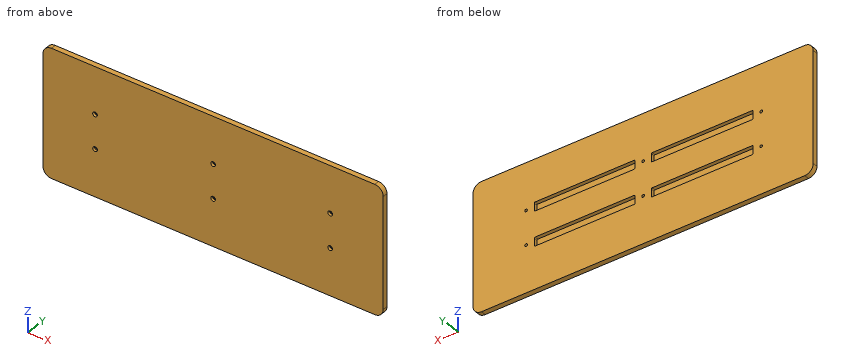
from build123d import *

# Parameters (mm, degrees)
IZIM1_W                     = 400
IZIM1_H                     = 150
Y_KSEKLIK_EKSTR_ZYON1_DEPTH = 6
IZIM2_W                     = 119.6
IZIM2_H                     = 10.4
IZIM2_W_2                   = 118.39
KES_EKSTR_ZYON1_DEPTH       = 4.4
RADYUS1_R                   = 10
IZIM3_R                     = 1.575
KES_EKSTR_ZYON2_DEPTH       = 7
IZIM4_R                     = 2.75
KES_EKSTR_ZYON3_DEPTH       = 2.89
RADYUS2_R                   = 1


with BuildPart() as part:
    # Çizim1 → Yükseklik-Ekstrüzyon1 (new body)
    with BuildSketch(Plane(origin=(0, 0, 0), x_dir=(1, 0, 0), z_dir=(0, 1, 0))):
        Rectangle(IZIM1_W, IZIM1_H)
    extrude(amount=-Y_KSEKLIK_EKSTR_ZYON1_DEPTH)

    # Çizim2 → Kes-Ekstrüzyon1 (cut)
    with BuildSketch(Plane(origin=(0, 0, 0), x_dir=(1, 0, 0), z_dir=(0, 1, 0))):
        with Locations((-69.4, 20.2)):
            Rectangle(IZIM2_W, IZIM2_H)
        with Locations((-69.4, -20.2)):
            Rectangle(IZIM2_W, IZIM2_H)
        with Locations((68.795, 20.2)):
            Rectangle(IZIM2_W_2, IZIM2_H)
        with Locations((68.795, -20.2)):
            Rectangle(IZIM2_W_2, IZIM2_H)
    extrude(amount=-KES_EKSTR_ZYON1_DEPTH, mode=Mode.SUBTRACT)

    # Radyus1
    radyus1_edges = [part.edges().sort_by_distance(p)[0] for p in [
        (200, -3, 75),
        (-200, -3, 75),
        (-200, -3, -75),
        (200, -3, -75),
    ]]
    fillet(radyus1_edges, radius=RADYUS1_R)

    # Çizim3 → Kes-Ekstrüzyon2 (cut, through all)
    with BuildSketch(Plane.XZ.offset(6)):
        with Locations((-138.8, 20)):
            Circle(IZIM3_R)
        with Locations((0, 20)):
            Circle(IZIM3_R)
        with Locations((137.59, 20)):
            Circle(IZIM3_R)
        with Locations((137.59, -20)):
            Circle(IZIM3_R)
        with Locations((0, -20)):
            Circle(IZIM3_R)
        with Locations((-138.8, -20)):
            Circle(IZIM3_R)
    extrude(amount=-KES_EKSTR_ZYON2_DEPTH, mode=Mode.SUBTRACT)

    # Çizim4 → Kes-Ekstrüzyon3 (cut)
    with BuildSketch(Plane.XZ.offset(6)):
        with Locations((-138.8, 20)):
            Circle(IZIM4_R)
        with Locations((0, 20)):
            Circle(IZIM4_R)
        with Locations((137.59, 20)):
            Circle(IZIM4_R)
        with Locations((137.59, -20)):
            Circle(IZIM4_R)
        with Locations((0, -20)):
            Circle(IZIM4_R)
        with Locations((-138.8, -20)):
            Circle(IZIM4_R)
    extrude(amount=-KES_EKSTR_ZYON3_DEPTH, mode=Mode.SUBTRACT)

    # Radyus2
    radyus2_edges = [part.edges().sort_by_distance(p)[0] for p in [
        (127.99, -2.2, -15),
        (9.6, -2.2, -15),
        (9.6, -2.2, -25.4),
        (127.99, -2.2, -25.4),
        (-9.6, -2.2, -25.4),
        (-9.6, -2.2, -15),
        (-129.2, -2.2, -15),
        (-129.2, -2.2, -25.4),
        (127.99, -2.2, 15),
        (127.99, -2.2, 25.4),
        (9.6, -2.2, 25.4),
        (9.6, -2.2, 15),
        (-9.6, -2.2, 15),
        (-9.6, -2.2, 25.4),
        (-129.2, -2.2, 25.4),
        (-129.2, -2.2, 15),
    ]]
    fillet(radyus2_edges, radius=RADYUS2_R)


solid = part.part
Read the model definition and answer for the solid it produces. Units are mm, in the model's axes. Give positions to 0.01 mm unless a question says otherwise; leave off trailing zeros. Write each loop counter-clockwise with the first axis right and the second up, starting at its lowest first coordinate (ties: lowest second). Pieces come first, ordered by that corner, then holes. Notation, with made-up numbers: (77, -4.75) -> (133, -4.75) arc R27 ccw to (133, 24.25) -> close; hole circle Ø3 at (53, 0.25). An arc over 180 degrees is marked (long way). Answer as a JSON object with one key per item and string values. Group by question number.
1) Find section B-B (y = -2.2). Count the separate pieces of the cut face and the enclosed holes in it, and give its area (3 significant figures).
2) Each of these flat-tipped pins is pushed along its axis until it touches: P1, Ø1.6, axis at x = 138.5, z = -21, coming from the -Y side; P2, Ø8.5, axis at x = -82.5, z = -19, coming from the +Y side; P3, Ø5, axis at x = -51.5, z = 21.5, coming from the +Y side. Where does it stop, or does it pass through?
3) Consider L1, parallel to Z at x = -138.8, y = -4.25; L2, parallel to Z at x = 137.59, y = -1.55 (3 decimals); L3, parallel to X at y = -3.7, z = -15.5. Determine where each line is inside the solid, lowest interval first. Write a range as from..to.
4) Find section A-A (x = -105.5). Write down the section's boundary in (y, z), and give its area (3 significant figures).
Values follow:
{
 "1": {"separate pieces": "1", "enclosed holes": "10", "area": "54,900 mm2"},
 "2": {"P1": "stops at y = -3.11", "P2": "stops at y = 0", "P3": "stops at y = -4.4"},
 "3": {"L1": "z = -75..-22.75, -17.25..17.25, 22.75..75", "L2": "z = -75..-21.575, -18.425..18.425, 21.575..75", "L3": "x = -200..-129.07, -9.73..9.73, 127.86..200"},
 "4": {"outline": "(-6, -75) -> (0, -75) -> (0, -25.4) -> (-4.4, -25.4) -> (-4.4, -15) -> (0, -15) -> (0, 15) -> (-4.4, 15) -> (-4.4, 25.4) -> (0, 25.4) -> (0, 75) -> (-6, 75) -> close", "area": "808 mm2"}
}
